Job drawing, mm, ordinate dimensions from the low corner. One solid piece. Coordinates: 2 decimals unless noted, no trailing zeros. Loops run counter-clockwise (first coordinate to the right, second up) from the corner with the lowest first, then second, coordinate; pieces in that order, holes last. Notation, with made-up numbers: (22.25, -36.75) -> (57.25, -36.75) arc R29 ccw to (57.25, -12.75) -> close; hole circle Ø7 at (4.25, -17). An arc over 180 degrees is marked (long way). Answer as CSV lines item,"result". Start each with the question number.
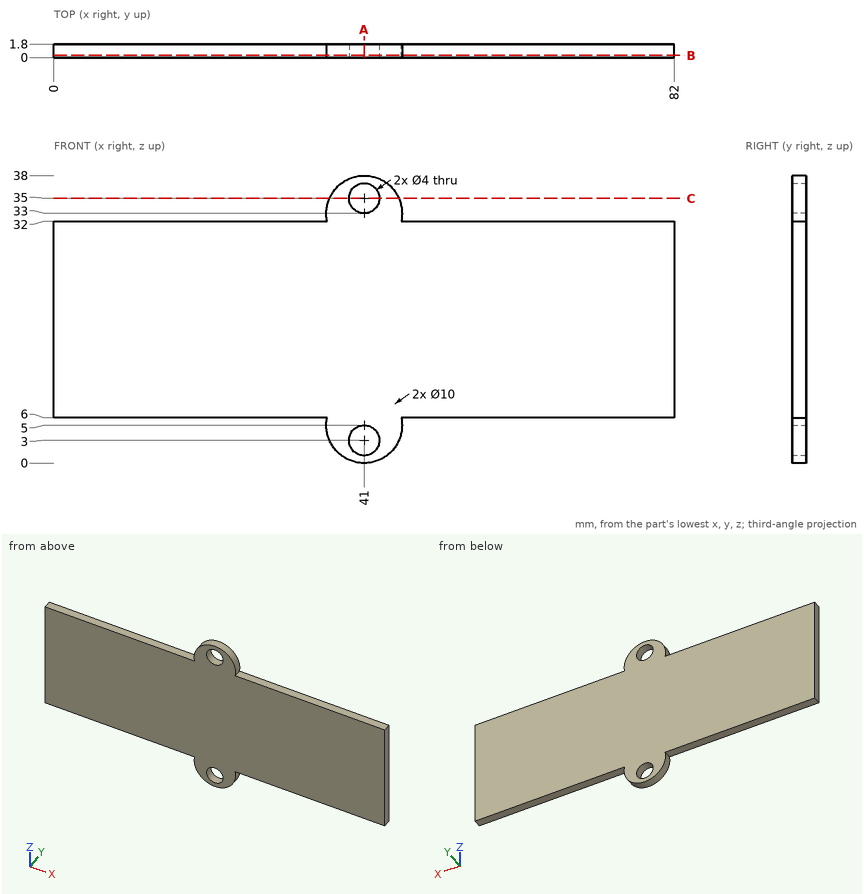
Q1. Saw through at C-C (z = 35). List the corners of the cut face in (x, y), and give its area (3 significant figures).
Q2. Saw through at B-B (y = 0.3). List the corners of the cut face in (x, z).
Q3. Pin check, flat tip, straight feed: pin 1 Ø1.5 at (x, z) = (73, 4) entering from -Y. Stop position of the tip, or through.
Q4. Saw through at A-A (x = 41). List the corners of the cut face in (y, z).
Q5. Probe probe 1 along Z at (x, y) = (7.5, 1.15); probe 2 along X at (y, z) = (0.7, 3); probe 3 along X at (y, z) = (1.5, 34). List the from-to ranges inside material, lowest first. Write a range as from..to.
Ans:
1,outline,"(36.42, 0) -> (39, 0) -> (39, 1.8) -> (36.42, 1.8) -> close; (43, 0) -> (45.58, 0) -> (45.58, 1.8) -> (43, 1.8) -> close"
1,area,"9.30 mm²"
2,outline,"(0, 6) -> (36.1, 6) arc R5 ccw (long way) to (45.9, 6) -> (82, 6) -> (82, 32) -> (45.9, 32) arc R5 ccw (long way) to (36.1, 32) -> (0, 32) -> close; hole circle Ø4 at (41, 3); hole circle Ø4 at (41, 35)"
3,pin 1,"passes through"
4,outline,"(0, 0) -> (1.8, 0) -> (1.8, 1) -> (0, 1) -> close; (0, 5) -> (1.8, 5) -> (1.8, 33) -> (0, 33) -> close; (0, 37) -> (1.8, 37) -> (1.8, 38) -> (0, 38) -> close"
5,probe 1,"z = 6..32"
5,probe 2,"x = 36.42..39, 43..45.58"
5,probe 3,"x = 36.1..39.27, 42.73..45.9"
